```python
from build123d import *

# Parameters (mm, degrees)
WYCI_GNI_CIE1_DEPTH        = 4
SFAZOWANIE1_SIZE           = 0.3
SZKIC3_R                   = 3.68172134
WYTNIJ_WYCI_GNI_CIE1_DEPTH = 2
WYTNIJ_WYCI_GNI_CIE1_DRAFT = -45
SFAZOWANIE2_SIZE           = 0.5


with BuildPart() as part:
    # Szkic1 → Obrót1 (revolve)
    with BuildSketch(Plane.XY, mode=Mode.PRIVATE) as obr_t1_sk:
        Polygon((0, 0), (-4, 0), (-4, 80), (-6.25, 80), (-6.25, 88), (0, 88), align=None)
    revolve(obr_t1_sk.sketch.rotate(Axis((0, 0, 0), (0, 1, 0)), 270), axis=Axis((0, 0, 0), (0, 1, 0)))

    # Szkic2 → Wyciągnięcie1 (cut)
    with BuildSketch(Plane(origin=(0, 88, 0), x_dir=(1, 0, 0), z_dir=(0, 1, 0))):
        Polygon((3.464101615, 0), (1.732050808, 3), (-1.732050808, 3), (-3.464101615, 0), (-1.732050808, -3), (1.732050808, -3), align=None)
    extrude(amount=-WYCI_GNI_CIE1_DEPTH, mode=Mode.SUBTRACT)

    # Sfazowanie1
    sfazowanie1_edges = [part.edges().sort_by_distance(p)[0] for p in [
        (0, 88, 6.25),
    ]]
    chamfer(sfazowanie1_edges, length=SFAZOWANIE1_SIZE)


with BuildPart() as wytnij_wyci_gni_cie1_tool:
    # Szkic3 → Wytnij-wyciągnięcie1 (with draft: the straight prism first)
    with BuildSketch(Plane(origin=(0, 88, 0), x_dir=(1, 0, 0), z_dir=(0, 1, 0))):
        Circle(SZKIC3_R)
    extrude(amount=-WYTNIJ_WYCI_GNI_CIE1_DEPTH)
    # Wytnij-wyciągnięcie1: the draft: its side faces are tilted about the plane it starts from
    wytnij_wyci_gni_cie1_sides = [wytnij_wyci_gni_cie1_tool.faces().sort_by_distance(p)[0] for p in [
        (-3.68172134, 87, 0),
    ]]
    draft(wytnij_wyci_gni_cie1_sides, Plane(origin=(0, 88, 0), x_dir=(1, 0, 0), z_dir=(0, 1, 0)), WYTNIJ_WYCI_GNI_CIE1_DRAFT)


with BuildPart() as part_1:
    add(part.part)

    # Wytnij-wyciągnięcie1: cut by wytnij_wyci_gni_cie1_tool
    add(wytnij_wyci_gni_cie1_tool.part, mode=Mode.SUBTRACT)

    # Sfazowanie2
    sfazowanie2_edges = [part_1.edges().sort_by_distance(p)[0] for p in [
        (0, 0, 4),
    ]]
    chamfer(sfazowanie2_edges, length=SFAZOWANIE2_SIZE)


solid = part_1.part
```
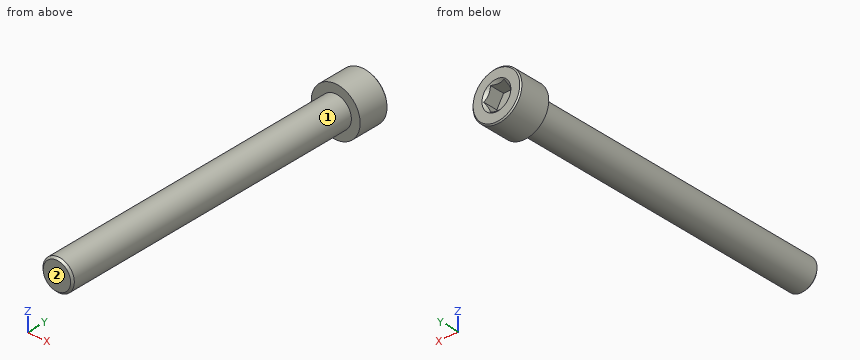
CAD build for the part. Positions are in the model's coordinates, mm. Face numbers are marked on the shaded views. A direction names the side the tool comes from. Round coordinates to 2 decimals unless told otherwise and drop trailing zeros. Write each loop counter-clockwise with the first axis right and the second up, starting at its lowest first coordinate (ties: lowest second). Pieces come first, ordered by that corner, then holes. Notation, with made-up numbers: M 10.25,5.5 L 14.25,5.5 A5 ccw 14.25,10.5 Z; hole C 17.25,-13 d10. An arc over 180 degrees is marked long. One line per question, with ' | ' between items.
1. Cut at B-B on y = 24. Write the cut outline in (x, z).
Working result:
outline: C 0,0 d8
2. Probe L1, parallel to Y at x = 1, z = -4.5; L2, parallel to X at y = 13.5, z = -2; L3, parallel to Z at x = -0.25, y = 35.5. List the from-to ranges inside material, lowest first. Write a range as from..to.
Working result:
L1: 80..88 | L2: -3.46..3.46 | L3: -3.99..3.99
3. Cut at A-A on x = 0. Write the cut outline in (y, z), and give its area (3 significant figures).
Working result:
outline: M 0,-3.5 L 0.5,-4 L 80,-4 L 80,-6.25 L 87.7,-6.25 L 88,-5.95 L 88,-3.68 L 87.32,-3 L 84,-3 L 84,3 L 87.32,3 L 88,3.68 L 88,5.95 L 87.7,6.25 L 80,6.25 L 80,4 L 0.5,4 L 0,3.5 Z | area: 715 mm2
4. Which spindle directions (+Z, -Z, +X, -X, +Y, -Y) get a long thin tool onto all of the face, cutting with end or side? Do the marked faces 1 and 2. Say none if no direction does.
Working result:
face 1: -Y | face 2: +Z, -Z, +X, -X, -Y
5. Pin check, flat tips, straight feed: pin 1 Ø4 at (y, z) = (74.5, 4) entering from -X; pin 2 Ø1.8 at (x, z) = (-1.5, -1) entering from +Y; pin 3 Ø2 at (x, z) = (0.5, 3) entering from -Y; pin 4 Ø1 at (y, z) = (72.5, -3) entering from -X. Stop position of each tip, or through.
Working result:
pin 1: x = -3.46 | pin 2: y = 84 | pin 3: y = 0 | pin 4: x = -3.12
